Build history of the part. All positions in model axes, mm. A direction names the side the tool comes from. Round coordinates to 2 decimals unless told otherwise and drop trailing zeros. Loops run counter-clockwise (first coordinate to the right, second up) from the corner with the lowest first, then second, coordinate; pieces in that order, holes last. Notation, with made-up numbers: M -5,81 L 38,81 A27 cw 38,100 Z; hole C -22,-5 d6. An arc over 180 degrees is marked long. One line per item, written item: value.
```python
from build123d import *

# Parameters (mm, degrees)
CYLINDER001_R               = 4.2
CYLINDER001_DEPTH           = 120
CYLINDER001_ROLL_ANGLE      = -89.998101
CYLINDER001_PITCH_ANGLE     = 89.45035
CYLINDER001_PLACEMENT_ANGLE = -89.998101
CYLINDER_R                  = 4.2
CYLINDER_DEPTH              = 120
CYLINDER_PITCH_ANGLE        = 90
CYLINDER008_R               = 2
CYLINDER008_DEPTH           = 80
ARRAY006_X_COUNT            = 3
ARRAY006_X_PITCH            = 45
CYLINDER010_R               = 2
CYLINDER010_DEPTH           = 80
ARRAY007_X_COUNT            = 3
ARRAY007_X_PITCH            = 45
CYLINDER009_R               = 7.7
CYLINDER009_DEPTH           = 24.4
CYLINDER009_PITCH_ANGLE     = 90
ARRAY005_X_COUNT            = 2
ARRAY005_X_PITCH            = 35.6
CYLINDER007_R               = 7.7
CYLINDER007_DEPTH           = 24.4
CYLINDER007_PITCH_ANGLE     = 90
ARRAY004_X_COUNT            = 2
ARRAY004_X_PITCH            = 35.6
BOX003_W                    = 40
BOX003_H                    = 38
BOX003_DEPTH                = 25
BOX002_W                    = 40
BOX002_H                    = 38
BOX002_DEPTH                = 25
BOX004_W                    = 110
BOX004_H                    = 100
BOX004_DEPTH                = 15


with BuildPart() as cylinder001:
    # Cylinder001 → Cylinder001 (new body)
    with BuildSketch(Plane.XY):
        Circle(CYLINDER001_R)
    extrude(amount=CYLINDER001_DEPTH)


with BuildPart() as cylinder001_1:
    # Cylinder001 roll: moved
    add(cylinder001.part.rotate(Axis((0, 0, 0), (1, 0, 0)), CYLINDER001_ROLL_ANGLE))


with BuildPart() as cylinder001_2:
    # Cylinder001 pitch: moved
    add(cylinder001_1.part.rotate(Axis((0, 0, 0), (0, 1, 0)), CYLINDER001_PITCH_ANGLE))


with BuildPart() as cylinder001_3:
    # Cylinder001 placement: moved
    add(cylinder001_2.part.moved(Location((-5, 80, 0))).rotate(Axis((-5, 80, 0), (0, 0, 1)), CYLINDER001_PLACEMENT_ANGLE))


with BuildPart() as ejes:
    # Cylinder → Cylinder (new body)
    with BuildSketch(Plane.XY):
        Circle(CYLINDER_R)
    extrude(amount=CYLINDER_DEPTH)


with BuildPart() as ejes_1:
    # Cylinder pitch: moved
    add(ejes.part.rotate(Axis((0, 0, 0), (0, 1, 0)), CYLINDER_PITCH_ANGLE))


with BuildPart() as ejes_2:
    # Cylinder placement: moved
    add(ejes_1.part.moved(Location((-5, 20, 0))))

    # Fusion001: union Cylinder001
    add(cylinder001_3.part)


with BuildPart() as array006:
    # Cylinder008 → Cylinder008 (new body)
    with BuildSketch(Plane(origin=(10, 6, -30), x_dir=(1, 0, 0), z_dir=(0, 0, 1))):
        Circle(CYLINDER008_R)
    extrude(amount=CYLINDER008_DEPTH)

    # Array006 X: Array006 ×3


with BuildPart() as array006_1:
    add(array006.part)
    with Locations(*[(i * ARRAY006_X_PITCH, 0, 0) for i in range(1, ARRAY006_X_COUNT)]):
        add(array006.part)


with BuildPart() as array007:
    # Cylinder010 → Cylinder010 (new body)
    with BuildSketch(Plane(origin=(10, 6, -30), x_dir=(1, 0, 0), z_dir=(0, 0, 1))):
        Circle(CYLINDER010_R)
    extrude(amount=CYLINDER010_DEPTH)

    # Array007 X: Array007 ×3


with BuildPart() as array007_1:
    add(array007.part)
    with Locations(*[(i * ARRAY007_X_PITCH, 0, 0) for i in range(1, ARRAY007_X_COUNT)]):
        add(array007.part)


with BuildPart() as array007_2:
    # Array007 placement: moved
    add(array007_1.part.moved(Location((0, 88, 0))))


with BuildPart() as array005:
    # Cylinder009 → Cylinder009 (new body)
    with BuildSketch(Plane.XY):
        Circle(CYLINDER009_R)
    extrude(amount=CYLINDER009_DEPTH)


with BuildPart() as array005_1:
    # Cylinder009 pitch: moved
    add(array005.part.rotate(Axis((0, 0, 0), (0, 1, 0)), CYLINDER009_PITCH_ANGLE))


with BuildPart() as array005_2:
    # Cylinder009 placement: moved
    add(array005_1.part.moved(Location((25, 80, 0))))

    # Array005 X: Array005 ×2


with BuildPart() as array005_3:
    add(array005_2.part)
    with Locations(*[(i * ARRAY005_X_PITCH, 0, 0) for i in range(1, ARRAY005_X_COUNT)]):
        add(array005_2.part)


with BuildPart() as obj1:
    # Cylinder007 → Cylinder007 (new body)
    with BuildSketch(Plane.XY):
        Circle(CYLINDER007_R)
    extrude(amount=CYLINDER007_DEPTH)


with BuildPart() as obj1_1:
    # Cylinder007 pitch: moved
    add(obj1.part.rotate(Axis((0, 0, 0), (0, 1, 0)), CYLINDER007_PITCH_ANGLE))


with BuildPart() as obj1_2:
    # Cylinder007 placement: moved
    add(obj1_1.part.moved(Location((25, 20, 0))))

    # Array004 X: obj1_2


with BuildPart() as obj1_3:
    add(obj1_2.part)
    with Locations(*[(i * ARRAY004_X_PITCH, 0, 0) for i in range(1, ARRAY004_X_COUNT)]):
        add(obj1_2.part)

    # Fusion005: union Array006, Array007, Array005
    add(array006_1.part)
    add(array007_2.part)
    add(array005_3.part)


with BuildPart() as cubo003:
    # Box003 → Box003 (new body)
    with BuildSketch(Plane(origin=(97, 31, -10), x_dir=(1, 0, 0), z_dir=(0, 0, 1))):
        with Locations((20, 19)):
            Rectangle(BOX003_W, BOX003_H)
    extrude(amount=BOX003_DEPTH)


with BuildPart() as fusion002:
    # Box002 → Box002 (new body)
    with BuildSketch(Plane(origin=(-27, 31, -10), x_dir=(1, 0, 0), z_dir=(0, 0, 1))):
        with Locations((20, 19)):
            Rectangle(BOX002_W, BOX002_H)
    extrude(amount=BOX002_DEPTH)

    # Fusion002: union Cubo003
    add(cubo003.part)


with BuildPart() as cut005:
    # Box004 → Box004 (new body)
    with BuildSketch(Plane.XY.offset(-15)):
        with Locations((55, 50)):
            Rectangle(BOX004_W, BOX004_H)
    extrude(amount=BOX004_DEPTH)

    # Cut: cut Fusion002
    add(fusion002.part, mode=Mode.SUBTRACT)

    # Cut003: cut obj1
    add(obj1_3.part, mode=Mode.SUBTRACT)

    # Cut005: cut Ejes
    add(ejes_2.part, mode=Mode.SUBTRACT)


solid = cut005.part
```
Item 1: Which spindle directions (+Z, -Z, +X, -X, +Y, -Y) get a long thin tool onto all of the face, cutting with end or side? Do faces 5 (the face through (103, 31, -5)), 6 (the face through (6, 69, -5)), 7 (the face through (37.03, 19.83, -7.7)). Say none if no direction does.
Check values:
face 5: +Z, +X
face 6: +Z, -X
face 7: +Z
Item 2: Wall check: line 1 along Y through (x, z) = (10, -5.75); line 2 along X through (y, z) = (6, -5.75); line 3 along Y through (x, z) = (55, -9.75). Give the ranges that are in metal, low to high.
Check values:
line 1: y = 0 to 4, 8 to 31, 69 to 92, 96 to 100
line 2: x = 0 to 8, 12 to 53, 57 to 98, 102 to 110
line 3: y = 0 to 4, 8 to 92, 96 to 100
Item 3: Slice it at D-D, the plane y = 20. Give the cut face in (x, z).
Check values:
outline: M 0,-15 L 110,-15 L 110,-4.2 L 85,-4.2 L 85,-7.7 L 60.6,-7.7 L 60.6,-4.2 L 49.4,-4.2 L 49.4,-7.7 L 25,-7.7 L 25,-4.2 L 0,-4.2 Z
Item 4: Pull direction X, two halves, no side cores. Call faces 1 (the face through (54.9, 19.9, -4.2)), 2 (the face through (49.4, 20, -5)), 3 (the face through (13, 50, -5)), 4 (the face through (85, 80, -5)): pulls with the +X half, pulls with the -X half, needs draft (parallel to the pull), parting line crosses it, or undercut.
Check values:
face 1: needs draft
face 2: undercut
face 3: pulls with the -X half
face 4: undercut
Item 5: Drop flat-ended pins along their axis: P1, Ø3, axis at x = 25, z = -3, coming from the -Y side; P2, Ø4, axis at x = 102, y = 49.5, coming from the +Z side; P3, Ø1, axis at y = 66.5, z = -5, coming from the -X side; P4, Ø4, axis at x = 77, y = 75.5, coming from the +Z side. Give the stop position or say it passes through.
Check values:
P1: stops at y = 0
P2: stops at z = -10
P3: stops at x = 13
P4: stops at z = -4.13
Item 6: Slice it at A-A, the plane y = 6. Give the cut face in (x, z).
Check values:
outline: M 0,-15 L 8,-15 L 8,0 L 0,0 Z; M 12,-15 L 53,-15 L 53,0 L 12,0 Z; M 57,-15 L 98,-15 L 98,0 L 57,0 Z; M 102,-15 L 110,-15 L 110,0 L 102,0 Z
Item 7: Slice it at B-B, the plane z = -6. Give the number of separate pieces and of enclosed holes in the cut face, and give its area (3 significant figures).
Check values:
separate pieces: 1
enclosed holes: 10
area: 8,990 mm2
